Geometry: see drawing. Coordinates: mm, zero at the bounding-box minimum. A direction names the side the tool comes from. Round coordinates to 2 decimals unless told otherwise and drop trailing zeros. Order: outer loops, then holes, each group sorted by start corner. A loop starts at its lowest first (then second) coordinate and runs counter-clockwise, first axis right, second up. Notation, with made-up numbers: (61.5, 18) -> (73.5, 18) arc R18 ccw to (73.5, 48) -> close; hole circle Ø7 at (-33.5, 83.25). An arc over 180 degrees is marked (long way). Put each result on its own line as item: value.
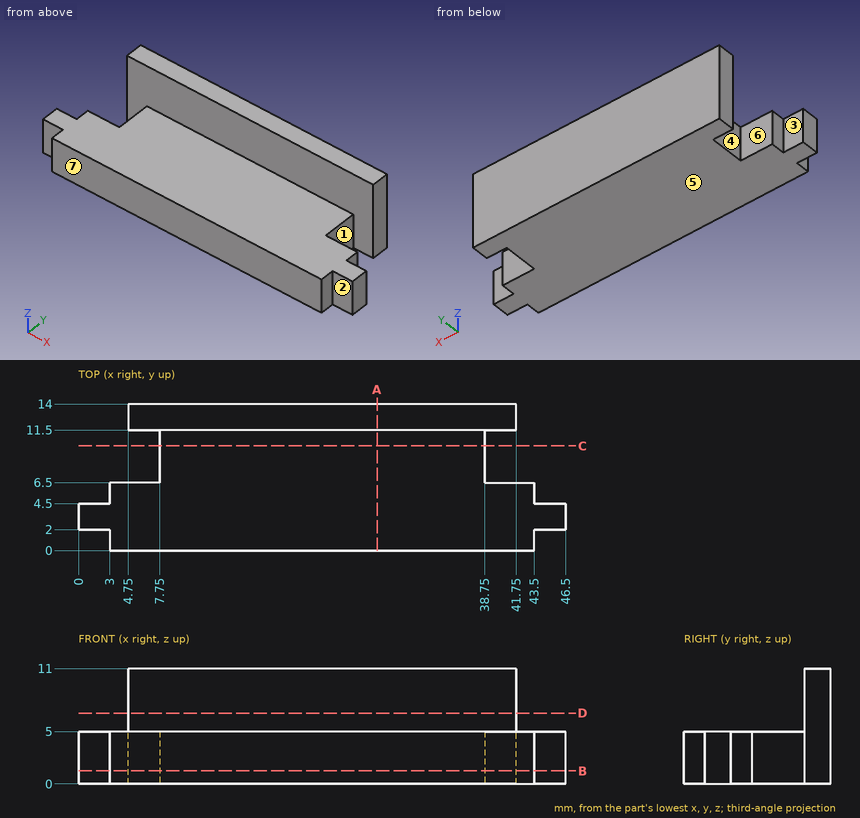
1. Contact query for flat-ended pins moving along their axis: P1, Ø3.5, axis at x = 45.5, z = 2.5, coming from the -Y side; P2, Ø4, axis at x = 9.5, y = 6.5, coming from the +Z side; P3, Ø3.5, axis at x = 44.5, z = 1.5, coming from the +Y side. Output: stop coordinate, or through.
Ans:
P1: y = 2
P2: z = 5
P3: y = 6.5
2. Cut plane D-D on z = 6.75. Return loops of the section in (x, y), and give its area (3 significant figures).
Ans:
outline: (4.75, 11.5) -> (41.75, 11.5) -> (41.75, 14) -> (4.75, 14) -> close
area: 92.5 mm²
3. Material intervals for probe 1 along Y at (x, z) = (5.5, 4); probe 2 along Y at (x, z) = (35, 7); probe 3 along X at (y, z) = (12.5, 4.25), sorted ascending.
Ans:
probe 1: 0 to 6.5, 11.5 to 14
probe 2: 11.5 to 14
probe 3: 4.75 to 41.75
4. Cut plane B-B on z = 1.25. Return loops of the section in (x, y).
Ans:
outline: (0, 2) -> (3, 2) -> (3, 0) -> (43.5, 0) -> (43.5, 2) -> (46.5, 2) -> (46.5, 4.5) -> (43.5, 4.5) -> (43.5, 6.5) -> (38.75, 6.5) -> (38.75, 11.5) -> (41.75, 11.5) -> (41.75, 14) -> (4.75, 14) -> (4.75, 11.5) -> (7.75, 11.5) -> (7.75, 6.5) -> (3, 6.5) -> (3, 4.5) -> (0, 4.5) -> close
5. Draft query along Y for the marked faces 5, 6 and 7. Return one class per face: +Y half, -Y half, draft (parallel to the pull), parting line (faces both ways), or undercut.
Ans:
face 5: draft
face 6: undercut
face 7: -Y half
6. Set-up query: the marked faces 1, 2, 3 and 4. Return all of +Z, -Z, +X, -X, +Y, -Y with unobstructed straight access to the full face (end or side cutting, diameter ignored); none if empty.
Ans:
face 1: +Z, -Z, +X
face 2: +Z, -Z, +X, -Y
face 3: +Z, -Z, -X, +Y
face 4: +Z, -Z, -X
7. Cut plane C-C on y = 10. Return loops of the section in (x, z), and give its area (3 significant figures).
Ans:
outline: (7.75, 0) -> (38.75, 0) -> (38.75, 5) -> (7.75, 5) -> close
area: 155 mm²
8. Cut plane A-A on x = 28.5. Return loops of the section in (y, z).
Ans:
outline: (0, 0) -> (14, 0) -> (14, 11) -> (11.5, 11) -> (11.5, 5) -> (0, 5) -> close
